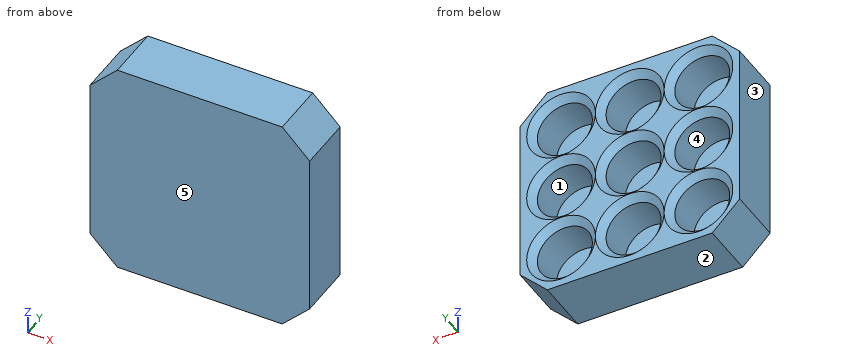
Autodesk Inventor part; units mm, degrees
ref_plane "YZ Plane" through (0, 0, 0) normal (1, 0, 0) x (0, 1, 0)
ref_plane "XZ Plane" through (0, 0, 0) normal (0, 1, 0) x (-1, 0, 0)
ref_plane "XY Plane" through (0, 0, 0) normal (0, 0, 1) x (1, 0, 0)
sketch "Esquisse1" plane through (0, 0, 0) normal (0, 1, 0) x (-1, 0, 0)
  line L0 (0, 0) -> (32, 0)
  line L1 (32, 0) -> (32, 32)
  line L2 (32, 32) -> (0, 32)
  line L3 (0, 32) -> (0, 0)
  dimension "d0" = 32
  dimension "d1" = 32
extrude "Extrusion1" add sketch "Esquisse1" along normal blind 8
sketch "Esquisse2" plane through (0, 8, 0) normal (0, 1, 0) x (1, 0, 0)
  line L0 (-32, 0) -> (-32, -32)
  line L1 (-32, -30) -> (12, -30)
  line L2 (-32, -2) -> (0.5255, -2)
  line L3 (-30, -30) -> (-30, -2)
  line L4 (-2, -30) -> (-2, -2)
  line L5 (0, -32) -> (0, 0)
  line L6 (-32, -32) -> (0, -32)
  line L7 (0, 0) -> (-32, 0)
  circle A0 centre (-26, -26) radius 4
  circle A1 centre (-26, -16) radius 4
  circle A2 centre (-26, -6) radius 4
  circle A3 centre (-16, -26) radius 4
  circle A4 centre (-16, -16) radius 4
  circle A5 centre (-16, -6) radius 4
  circle A6 centre (-6, -26) radius 4
  circle A7 centre (-6, -16) radius 4
  circle A8 centre (-6, -6) radius 4
  dimension "d4" = 2
  dimension "d5" = 2
  dimension "d6" = 2
  dimension "d7" = 2
  dimension "d18" = 8
  dimension "d19" = 8
  dimension "d20" = 8
  dimension "d21" = 8
  dimension "d22" = 8
  dimension "d23" = 8
  dimension "d24" = 8
  dimension "d25" = 8
  dimension "d26" = 8
  dimension "d27" = 4
  dimension "d28" = 4
  dimension "d29" = 4
  dimension "d30" = 4
  dimension "d31" = 4
  dimension "d32" = 4
  dimension "d33" = 4
  dimension "d34" = 4
  dimension "d35" = 10
  dimension "d36" = 4
  dimension "d37" = 4
  dimension "d38" = 4
  dimension "d39" = 10
  dimension "d40" = 10
  dimension "d41" = 10
  dimension "d42" = 10
  dimension "d43" = 10
  dimension "d44" = 10
  dimension "d45" = 10
extrude "Extrusion2" cut sketch "Esquisse2" against normal blind 6 contours A1 | A3 | A7 | A5 | A2 | A0 | A8 | A6 | A4
chamfer "Chanfrein1" distance 4 angle 45 4 edges at (0, 4, 32) (0, 4, 0) (-32, 4, 0) (-32, 4, 32)
chamfer "Chanfrein2" distance 1 angle 45 9 edges at (-30, 8, 26) (-30, 8, 16) (-30, 8, 6) (-20, 8, 6) (-20, 8, 16) (-20, 8, 26) (-10, 8, 16) (-10, 8, 26) (-10, 8, 6)
properties part number "Plateau"
CAD build for the part. Positions are in the model's coordinates, mm. Face numbers are marked on the shaded views. A direction names the side the tool comes from. Give positions to 0.01 mm unless a question says otherwise; leave off trailing zeros. Write each loop counter-clockwise with the first axis right and the second up, starting at its lowest first coordinate (ties: lowest second). Pieces come first, ordered by that corner, then holes. Notation, with made-up numbers: M 79.5,71.25 L 108.5,71.25 A20 cw 108.5,95.25 Z; hole C -12.5,-9.75 d8. An arc over 180 degrees is marked long. Return JSON: item names as keys, results as strings. Group by question number.
(1) 3-axis set-ups, long thin cutter, end or side, ignore diameter. For the marked faces 4 and 5: which of +Z, -Z, +X, -X, +Y, -Y reach the whole face in a straight line?
(2) Flat gauge pins, fed straight in: pin 1 Ø5 at (x, z) = (-6, 16) entering from +Y; pin 2 Ø9 at (x, z) = (-26, 6) entering from +Y; pin 3 Ø4 at (x, z) = (-17.5, 27.5) entering from +Y. Where does each tip first touch, or does it go through?
(3) Band-saw the part on D-D (y = 0.5). Give the cut face in (x, z).
(4) Drill centre lines: L1, parallel to Z at x = -16, y = 5; L2, parallel to X at y = 4.45, z = 6; L3, parallel to X at y = 3.75, z = 28. Where is each one in solid material? Low to high. Write a range as [from, to].
(5) Band-saw the part on A-A (y = 5). State how many separate pieces and enclosed holes the cut face has, and give its area (3 significant figures).
(6) Mould opens along Z. For the marked faces 1, 2 and 3 say: pulls with the +Z half, pulls with the -Z half, needs draft (parallel to the pull), parting line crosses it, or undercut.
Entries:
{
 "1": {"face 4": "+Y", "face 5": "+Z, -Z, +X, -X, -Y"},
 "2": {"pin 1": "stops at y = 2", "pin 2": "stops at y = 7.5", "pin 3": "stops at y = 7.12"},
 "3": {"outline": "M -32,4 L -28,0 L -4,0 L 0,4 L 0,28 L -4,32 L -28,32 L -32,28 Z"},
 "4": {"L1": "z = [0, 2], [10, 12], [20, 22], [30, 32]", "L2": "x = [-32, -30], [-22, -20], [-12, -10], [-2, 0]", "L3": "x = [-32, -29.46], [-22.54, -19.46], [-12.54, -9.46], [-2.54, 0]"},
 "5": {"separate pieces": "1", "enclosed holes": "9", "area": "540 mm^2"},
 "6": {"face 1": "undercut", "face 2": "pulls with the -Z half", "face 3": "needs draft"}
}
